from build123d import *

# Parameters (mm, degrees)
BOSS_EXTRUDE4_DEPTH  = 4
SKETCH5_W            = 74
SKETCH5_H            = 8
BOSS_EXTRUDE5_DEPTH  = 30
SKETCH6_W            = 4
SKETCH6_H            = 36
BOSS_EXTRUDE6_DEPTH  = 18
CUT_EXTRUDE2_DEPTH   = 18
SKETCH9_W            = 30
SKETCH9_H            = 30
BOSS_EXTRUDE11_DEPTH = 6
SKETCH10_R           = 8
CUT_EXTRUDE3_DEPTH   = 50
CUT_EXTRUDE4_DEPTH   = 8
CUT_EXTRUDE5_DEPTH   = 8


with BuildPart() as part:
    # Sketch1 → Boss-Extrude4 (new, symmetric)
    with BuildSketch(Plane.XY):
        Polygon((-74, 0), (-74, 41), (-61, 54), (-13, 54), (0, 41), (0, 0), align=None)
    extrude(amount=BOSS_EXTRUDE4_DEPTH, both=True)

    # Sketch5 → Boss-Extrude5 (add)
    with BuildSketch(Plane.XY.offset(4)):
        with Locations((-37, 4)):
            Rectangle(SKETCH5_W, SKETCH5_H)
    extrude(amount=BOSS_EXTRUDE5_DEPTH)

    # Sketch6 → Boss-Extrude6 (add)
    with BuildSketch(Plane.XY):
        with Locations((-63, 26)):
            Rectangle(SKETCH6_W, SKETCH6_H)
        with Locations((-11, 26)):
            Rectangle(SKETCH6_W, SKETCH6_H)
    extrude(amount=BOSS_EXTRUDE6_DEPTH)

    # Sketch8 → Cut-Extrude2 (cut)
    with BuildSketch(Plane(origin=(0, 8, 0), x_dir=(1, 0, 0), z_dir=(0, 1, 0))):
        Polygon((-74, -28), (-67.996452301, -34), (-74, -34), align=None)
        Polygon((0, -34), (-6, -34), (0, -28), align=None)
    extrude(amount=-CUT_EXTRUDE2_DEPTH, mode=Mode.SUBTRACT)

    # Sketch9 → Boss-Extrude11 (add)
    with BuildSketch(Plane(origin=(0, 8, 0), x_dir=(1, 0, 0), z_dir=(0, 1, 0))):
        with Locations((-37, -19)):
            Rectangle(SKETCH9_W, SKETCH9_H)
    extrude(amount=BOSS_EXTRUDE11_DEPTH)

    # Sketch10 → Cut-Extrude3 (cut)
    with BuildSketch(Plane(origin=(0, 14, 0), x_dir=(1, 0, 0), z_dir=(0, 1, 0))):
        with Locations(Location((-37, -23, 0), (0, 0, 270))):
            Circle(SKETCH10_R)
    extrude(amount=-CUT_EXTRUDE3_DEPTH, mode=Mode.SUBTRACT)

    # Sketch11 → Cut-Extrude4 (cut)
    with BuildSketch(Plane(origin=(-9, 0, 0), x_dir=(0, 0, -1), z_dir=(1, 0, 0))):
        Polygon((-4, 44), (-18, 8), (-18, 44), align=None)
    extrude(amount=-CUT_EXTRUDE4_DEPTH, mode=Mode.SUBTRACT)

    # Sketch12 → Cut-Extrude5 (cut)
    with BuildSketch(Plane(origin=(-61, 0, 0), x_dir=(0, 0, -1), z_dir=(1, 0, 0))):
        Polygon((-4, 44), (-18, 8), (-18, 44), align=None)
    extrude(amount=-CUT_EXTRUDE5_DEPTH, mode=Mode.SUBTRACT)


solid = part.part
The listing builds one solid part. Answer for the finished solid, in the listing's coordinates (mm). A direction names the side the tool comes from. Give positions to 0.01 mm unless a question says otherwise; leave off trailing zeros. Loops run counter-clockwise (first coordinate to the right, second up) from the corner with the lowest first, then second, coordinate; pieces in that order, holes last. Notation, with made-up numbers: (-28.75, -2.75) - (2.25, -2.75) arc R15 cw to (2.25, 19.25) - close; hole circle Ø8 at (-4.75, 8.25). An arc over 180 degrees is marked (long way). Use one line per item in the form item = value.
1. Find the intervals of material crossed by line 1 along X through (y, z) = (13.5, 12.5); line 2 along X through (y, z) = (5.5, 23); line 3 along Y through (x, z) = (-47.5, 16), in increasing order. Write a range as [from, to].
Calculated:
line_1 = [-65, -61], [-52, -22], [-13, -9]
line_2 = [-74, -45], [-29, 0]
line_3 = [0, 14]
2. Section B-B on x = -37 is taken. Give the vertices of the cut face in (y, z).
Calculated:
outline = (0, -4) - (54, -4) - (54, 4) - (14, 4) - (14, 15) - (0, 15) - close; (0, 31) - (14, 31) - (14, 34) - (0, 34) - close
3. Which of the six approach directions +Z, -Z, +X, -X, +Y, -Y give full straight-line access (tool end or side, diameter ignored) to faces 4 (the face through (-63, 8, 19)), 5 (the face through (-65, 22, 9)), 6 (the face through (-9, 22, 9)), 7 (the face through (-74, 11, 1)), 8 (the face through (-37, 6, 34))?
Calculated:
face_4 = +Z, +Y
face_5 = +Z, -X, +Y
face_6 = +Z, +X, +Y
face_7 = +Z, -Z, -X, +Y, -Y
face_8 = +Z, +X, -X, +Y, -Y
4. The mould has two halves that part along X. Classify faces 1 (the face through (-37, 54, 0)), 2 (the face through (-41, 14, 15)), 3 (the face through (-71, 4, 31)): pulls with the +X half, pulls with the -X half, needs draft (parallel to the pull), parting line crosses it, or undercut.
Calculated:
face_1 = needs draft
face_2 = undercut
face_3 = pulls with the -X half
5. Section C-C on y = 10 is taken. Give the vertices of the cut face in (x, z), then the cut area to 3 significant figures.
Calculated:
outline = (-74, -4) - (0, -4) - (0, 4) - (-9, 4) - (-9, 17.22) - (-13, 17.22) - (-13, 4) - (-22, 4) - (-22, 34) - (-52, 34) - (-52, 4) - (-61, 4) - (-61, 17.22) - (-65, 17.22) - (-65, 4) - (-74, 4) - close; hole circle Ø16 at (-37, 23)
area = 1,400 mm^2
6. Section D-D on z = 11 is taken. Give the vertices of the cut face in (x, y).
Calculated:
outline = (-74, 0) - (0, 0) - (0, 8) - (-9, 8) - (-9, 26) - (-13, 26) - (-13, 8) - (-22, 8) - (-22, 14) - (-52, 14) - (-52, 8) - (-61, 8) - (-61, 26) - (-65, 26) - (-65, 8) - (-74, 8) - close
7. Given pin 1 Ø4 at (y, z) = (28.5, 12) entering from +X; pin 2 Ø12 at (x, y) = (-28, 21.5) entering from +Z; pin 3 Ø3 at (y, z) = (12.5, 16) entering from -X; pin 4 Ø13 at (x, z) = (-37, 23) entering from -Y, each flat-ended and moving along its own axis, determine where each tip first touches the part or whether it passes through.
Calculated:
pin_1 = -9
pin_2 = 4
pin_3 = -65
pin_4 = through
8. Section A-A on z = 23 is taken. Give the vertices of the cut face in (x, y).
Calculated:
outline = (-74, 0) - (-45, 0) - (-45, 14) - (-52, 14) - (-52, 8) - (-74, 8) - close; (-29, 0) - (0, 0) - (0, 8) - (-22, 8) - (-22, 14) - (-29, 14) - close
